The listing builds one solid part. Answer for the finished solid, in the listing's coordinates (mm). A direction names the side the tool comes from. Round coordinates to 2 decimals unless told otherwise and drop trailing zeros. Write each loop counter-clockwise with the first axis right and the second up, starting at its lowest first coordinate (ties: lowest second). Pieces come first, ordered by that corner, then holes.
from build123d import *

# Parameters (mm, degrees)
SKETCH1_R           = 7.5
BOSS_EXTRUDE1_DEPTH = 10
SKETCH2_R           = 4
BOSS_EXTRUDE2_DEPTH = 20
SKETCH3_R           = 5
BOSS_EXTRUDE3_DEPTH = 15
CUT_EXTRUDE1_DEPTH  = 7


with BuildPart() as part:
    # Sketch1 → Boss-Extrude1 (new body)
    with BuildSketch(Plane.XY):
        Circle(SKETCH1_R)
    extrude(amount=BOSS_EXTRUDE1_DEPTH)

    # Sketch2 → Boss-Extrude2 (add)
    with BuildSketch(Plane(origin=(0, 0, 0), x_dir=(-1, 0, 0), z_dir=(0, 0, -1))):
        Circle(SKETCH2_R)
    extrude(amount=BOSS_EXTRUDE2_DEPTH)

    # Sketch3 → Boss-Extrude3 (add)
    with BuildSketch(Plane(origin=(0, 0, -20), x_dir=(-1, 0, 0), z_dir=(0, 0, -1))):
        Circle(SKETCH3_R)
    extrude(amount=BOSS_EXTRUDE3_DEPTH)

    # Sketch4 → Cut-Extrude1 (cut)
    with BuildSketch(Plane.XY.offset(10)):
        Polygon((2.886751346, 5), (-2.886751346, 5), (-5.773502692, 0), (-2.886751346, -5), (2.886751346, -5), (5.773502692, 0), align=None)
    extrude(amount=-CUT_EXTRUDE1_DEPTH, mode=Mode.SUBTRACT)


solid = part.part
1. Section D-D on z = -29 is taken. Determine the outline of the cut face in (x, y), plus the area to 3 significant figures.
Geometry says:
outline: circle Ø10 at (0, 0)
area: 78.5 mm2
2. Straight lines are drawn through the part: line 1 along Z through (x, y) = (-0.25, -4.25); line 2 along Z through (x, y) = (-1, -6); line 3 along Z through (x, y) = (-1.25, -3.5). For each, find the intervals that lie inside material, in ascending order.
Geometry says:
line 1: z = -35 to -20, 0 to 3
line 2: z = 0 to 10
line 3: z = -35 to 3
3. A tool of negligible diameter and unlimited length cuts with its end or side. For faces 5 (the face through (5, 2, 10)), 6 (the face through (0.867, -3.905, -9.86)), 7 (the face through (4.31, -2.535, 6.549)), 8 (the face through (1.08, -4.88, -27.4)), from which of +Z, -Z, +X, -X, +Y, -Y can it reach the whole face along a straight path? Write none if from no direction.
Geometry says:
face 5: +Z, +X, -X, +Y, -Y
face 6: none
face 7: +Z
face 8: -Z
4. Section C-C on y = -6 is taken. Determine the outline of the cut face in (x, z).
Geometry says:
outline: (-4.5, 0) - (4.5, 0) - (4.5, 10) - (-4.5, 10) - close
5. For a pull along Z with two mould halves and no side action, classify faces 1 (the face through (3, -3, 0)), 2 (the face through (0, 0, -35)), 3 (the face through (0, 0, 3)), 4 (the face through (-4.35, -2.465, 6.549)) as released by +Z, released by -Z, zero draft, split by the parting line, or undercut.
Geometry says:
face 1: undercut
face 2: released by -Z
face 3: released by +Z
face 4: zero draft
6. Given pin 1 (3 mm diameter, centred on y = -1, z = -7.5, fed in from +X); pin 2 (6 mm diameter, centred on x = -3.5, z = -28, fed in from -Y); pin 3 (6 mm diameter, centred on y = -1.5, z = -28, fed in from -X), each flat-ended and moving along its own axis, determine where each tip first touches the part or whether it passes through.
Geometry says:
pin 1: stops at x = 4
pin 2: stops at y = -4.97
pin 3: stops at x = -5
7. Section A-A on z = 6 is taken. Determine the outline of the cut face in (x, y), plus the area to 3 significant figures.
Geometry says:
outline: circle Ø15 at (0, 0); hole (-5.77, 0) - (-2.89, -5) - (2.89, -5) - (5.77, 0) - (2.89, 5) - (-2.89, 5) - close
area: 90.1 mm2
8. Section B-B on x = 0 is taken. Determine the outline of the cut face in (y, z), plus the area to 3 significant figures.
Geometry says:
outline: (-7.5, 0) - (-4, 0) - (-4, -20) - (-5, -20) - (-5, -35) - (5, -35) - (5, -20) - (4, -20) - (4, 0) - (7.5, 0) - (7.5, 10) - (5, 10) - (5, 3) - (-5, 3) - (-5, 10) - (-7.5, 10) - close
area: 390 mm2
